Verification items for the finished model (mm, model axes). A direction names the side the tool comes from. Round coordinates to 2 decimals unless told otherwise and drop trailing zeros. Order: outer loops, then holes, each group sorted by start corner. A loop starts at its lowest first (then second) coordinate and runs counter-clockwise, first axis right, second up. Notation, with made-up numbers: M 14,-10.75 L 44,-10.75 A20 ccw 44,26.25 Z; hole C 70.25,38.5 d3. An arc over 180 degrees is marked long. One line per item, written item: value. Start each with the question number.
Solid Edge part; units mm, degrees
sketch "Sketch1" plane through (0, 0, 0) normal (0, -1, 0) x (1, 0, 0)
  line L0 (-122.1808, 13.3262) -> (-52.1808, 13.3262)
  line L1 (-52.1808, 13.3262) -> (-52.1808, 83.3262)
  line L2 (-52.1808, 83.3262) -> (-122.1808, 83.3262)
  line L3 (-122.1808, 83.3262) -> (-122.1808, 13.3262)
  line L4 (-118.1808, 17.3262) -> (-56.1808, 17.3262)
  line L5 (-56.1808, 17.3262) -> (-56.1808, 79.3262)
  line L6 (-56.1808, 79.3262) -> (-118.1808, 79.3262)
  line L7 (-118.1808, 79.3262) -> (-118.1808, 17.3262)
  dimension "D1" = 122.1808
  dimension "D2" = 52.1808
  dimension "D3" = 122.1808
extrude "Protrusion1" add sketch "Sketch1" against normal blind 1940
sketch "Sketch2" plane through (-87.1808, 1079, 13.3262) normal (0, 0, -1) x (0, -1, 0)
  circle A0 centre (-811, 0) radius 6.1
  circle A1 centre (-841, 0) radius 6.1
  circle A2 centre (1059, 0) radius 6.1
  dimension "D1" = 1059
  dimension "D2" = 841
extrude "Cutout1" cut sketch "Sketch2" against normal through all
sketch "Sketch3" plane through (-52.1808, 1079, 63.3262) normal (1, 0, 0) x (0, -1, 0)
  line L0 (1034, -16) -> (1079, -16)
  line L1 (1079, -16) -> (1079, 46)
  line L2 (1079, 46) -> (1034, 46)
  line L3 (1034, 46) -> (1034, -16)
  line L4 (-861, -16) -> (-806, -16)
  line L5 (-806, -16) -> (-806, 46)
  line L6 (-806, 46) -> (-861, 46)
  line L7 (-861, 46) -> (-861, -16)
  dimension "D1" = 806
  dimension "D2" = 806
  dimension "D3" = 1034
  dimension "D4" = 1034
extrude "Cutout2" cut sketch "Sketch3" against normal up to next
sketch "Sketch4" plane through (-92.1808, 1005.1, 13.3262) normal (0, 0, -1) x (0, -1, 0)
  line L0 (-934.9, 30) -> (-902.95, 30)
  line L1 (-902.95, 30) -> (-934.9, 0.2062)
  line L2 (-934.9, 0.2062) -> (-934.9, 30)
  dimension "D1" = 934.9
extrude "Cutout3" cut sketch "Sketch4" against normal through all
sketch "Sketch5" plane through (-92.1808, 1005.1, 13.3262) normal (0, 0, -1) x (0, 1, 0)
  line L0 (-1005.1, -29) -> (-1004.2609, -30)
  line L1 (-1004.2609, -30) -> (-1005.1, -30)
  line L2 (-1005.1, -30) -> (-1005.1, -29)
  dimension "D1" = 1005.1
extrude "Cutout4" cut sketch "Sketch5" against normal through all
sketch "Sketch6" plane through (-122.1808, 957.9195, 48.3262) normal (-1, 0, 0) x (0, -1, 0)
  line L0 (-982.0805, -31) -> (-872.0805, -31)
  line L1 (-872.0805, -31) -> (-872.0805, 31)
  line L2 (-872.0805, 31) -> (-982.0805, 31)
  line L3 (-982.0805, 31) -> (-982.0805, -31)
  dimension "D1" = 982.0805
  dimension "D2" = 872.0805
extrude "Cutout5" cut sketch "Sketch6" against normal up to next
sketch "Sketch7" plane through (-122.1808, 957.9195, 48.3262) normal (-1, 0, 0) x (0, 1, 0)
  line L0 (-957.9195, -31) -> (-887.9195, -31)
  line L1 (-887.9195, -31) -> (-887.9195, 31)
  line L2 (-887.9195, 31) -> (-957.9195, 31)
  line L3 (-957.9195, 31) -> (-957.9195, -31)
  dimension "D1" = 957.9195
  dimension "D2" = 887.9195
extrude "Cutout6" cut sketch "Sketch7" against normal up to next
fillet "Round1" radius 5 4 edges at (-54.1808, 45, 79.3262) (-54.1808, 45, 17.3262) (-54.1808, 1885, 79.3262) (-54.1808, 1885, 17.3262)
properties material "Aluminum, 6061-T6"
1. Draft check along Z on faces 1 (the face through (-52.181, 956, 48)), 2 (the face through (-88, 984, 17.326)), 3 (the face through (-88, 956, 13.326)), 4 (the face through (-87, 984, 79.326)). Enter one of: released by +Z, released by -Z, zero draft, split by the parting line, or undercut.
2. Section check B-B (x = -106). Record the cut outline in (y, z), and give its area (3 significant figures).
3. Section check A-A (y = 1228). Record the cut outline in (x, z).
4. Depth check by flat-ended pin: pin 1 (1.2 mm diameter, centred on x = -55, z = 58, fed in from -Y); pin 2 (2 mm diameter, centred on x = -120, z = 50.5, fed in from -Y); pin 3 (2 mm diameter, centred on x = -54.5, z = 45.5, fed in from +Y). Enter the tip coordinate at first touch or a pass-through.
5. Tool access check on faces 5 (the face through (-122.181, 941, 49)), 6 (the face through (-56.181, 952, 48)). Record the directions out of +Z, -Z, +X, -X, +Y, -Y that give a thin tool (end or side, any length) a straight path to the whole face; none if there is none.
6. Scan lines: line 1 along X through (y, z) = (1151, 70); line 2 along Z through (x, y) = (-109.5, 539); line 3 along X through (y, z) = (20, 81.1). Record each from-to range of solid material in increasing order.
Geometry check:
1. face 1: zero draft
1. face 2: undercut
1. face 3: released by -Z
1. face 4: undercut
2. outline: M 0,13.33 L 1925.4,13.33 L 1925.4,17.33 L 0,17.33 Z; M 0,79.33 L 1925.4,79.33 L 1925.4,83.33 L 0,83.33 Z
2. area: 15,400 mm²
3. outline: M -122.18,13.33 L -52.18,13.33 L -52.18,83.33 L -122.18,83.33 Z; hole M -118.18,17.33 L -56.18,17.33 L -56.18,79.33 L -118.18,79.33 Z
4. pin 1: stops at y = 45
4. pin 2: stops at y = 70
4. pin 3: stops at y = 1885
5. face 5: +Z, -Z, -X, +Y, -Y
5. face 6: +Y, -Y
6. line 1: x = -122.18 to -118.18, -56.18 to -52.18
6. line 2: z = 13.33 to 17.33, 79.33 to 83.33
6. line 3: x = -122.18 to -93.28, -81.08 to -52.18
